from build123d import *

# Parameters (mm, degrees)
SKETCH1_R                       = 12.7
BOSS_EXTRUDE1_DEPTH             = 80
TAP_DRILL_FOR_1_4_20_TAP1_D     = 5.1054
TAP_DRILL_FOR_1_4_20_TAP1_DEPTH = 7.62
TAP_DRILL_FOR_1_4_20_TAP1_TIP   = 1.533816902
TAP_DRILL_FOR_1_4_20_TAP2_D     = 5.1054
TAP_DRILL_FOR_1_4_20_TAP2_DEPTH = 7.62
TAP_DRILL_FOR_1_4_20_TAP2_TIP   = 1.533816902


with BuildPart() as part:
    # Sketch1 → Boss-Extrude1 (new body)
    with BuildSketch(Plane(origin=(0, 0, 0), x_dir=(1, 0, 0), z_dir=(0, 1, 0))):
        with Locations(Location((0, 0, 0), (0, 0, 270))):
            Circle(SKETCH1_R)
    extrude(amount=BOSS_EXTRUDE1_DEPTH)

    # Tap Drill for 1/4-20 Tap1
    with Locations(Plane.XZ):
        with Locations((0, 0)):
            Hole(TAP_DRILL_FOR_1_4_20_TAP1_D / 2, depth=TAP_DRILL_FOR_1_4_20_TAP1_DEPTH)
            with Locations((0, 0, -(TAP_DRILL_FOR_1_4_20_TAP1_DEPTH + TAP_DRILL_FOR_1_4_20_TAP1_TIP / 2))):  # 118° drill point
                Cone(0, TAP_DRILL_FOR_1_4_20_TAP1_D / 2, TAP_DRILL_FOR_1_4_20_TAP1_TIP, mode=Mode.SUBTRACT)

    # Tap Drill for 1/4-20 Tap2
    with Locations(Plane(origin=(0, 80, 0), x_dir=(1, 0, 0), z_dir=(0, 1, 0))):
        with Locations((0, 0)):
            Hole(TAP_DRILL_FOR_1_4_20_TAP2_D / 2, depth=TAP_DRILL_FOR_1_4_20_TAP2_DEPTH)
            with Locations((0, 0, -(TAP_DRILL_FOR_1_4_20_TAP2_DEPTH + TAP_DRILL_FOR_1_4_20_TAP2_TIP / 2))):  # 118° drill point
                Cone(0, TAP_DRILL_FOR_1_4_20_TAP2_D / 2, TAP_DRILL_FOR_1_4_20_TAP2_TIP, mode=Mode.SUBTRACT)


solid = part.part
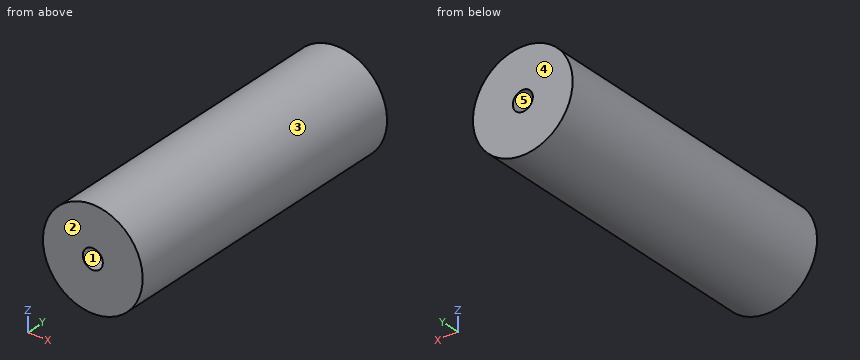
Verification items for the finished model (mm, model axes). Face numbers are marked on the shaded views. A direction names the side the tool comes from. Give positions to 0.01 mm unless a question says otherwise; leave off trailing zeros. Order: outer loops, then holes, each group sorted by start corner. A loop starts at its lowest first (then second) coordinate and runs counter-clockwise, first axis right, second up. Notation, with made-up numbers: M -6.5,84 L 8.5,84 A25 cw 8.5,103 Z; hole C 5.5,68.5 d6. An arc over 180 degrees is marked long. Use one line per item in the form item = value. Start each with the question number.
Q1. Access from +Z, -Z, +X, -X, +Y, -Y to the whole of each face (thin tool, end or side, straight path). Record for the marked faces 1 and 2.
Q2. Section check C-C (z = -10.75). Enter the section's corners in (x, y).
Q3. Go/stop test with flat-tipped pins: pin 1 Ø3 at (x, y) = (3, 55.5) entering from -Z; pin 2 Ø4 at (x, y) = (-9.5, 41) entering from -Z; pin 3 Ø12 at (y, z) = (47, 7.5) entering from -X. Record where each tip stops, or that it passes through.
Q4. Section check A-A (y = 64). Enter the section's corners in (x, z), then the cut area to 3 significant figures.
Q5. Section check B-B (x = -10.25). Enter the section's corners in (y, z), then the cut area to 3 significant figures.
Q6. Scan lines: line 1 along X through (y, z) = (4.5, 0); line 2 along Z through (x, y) = (-1, 74.5); line 3 along Z through (x, y) = (2.75, 21.5). Record each from-to range of solid material in increasing order. Write a range as [from, to].
Q7. Mould release check, pull along X, two halves, no side actions. Record for the marked faces 3, 4 and 5: +X half, -X half, draft (parallel to the pull), parting line (faces both ways), or undercut.
Evaluation:
q1.face_1 = -Y
q1.face_2 = +Z, -Z, +X, -X, -Y
q2.outline = M -6.76,0 L 6.76,0 L 6.76,80 L -6.76,80 Z
q3.pin_1 = -12.61
q3.pin_2 = -10.25
q3.pin_3 = -12.61
q4.outline = C 0,0 d25.4
q4.area = 507 mm2
q5.outline = M 0,-7.5 L 80,-7.5 L 80,7.5 L 0,7.5 Z
q5.area = 1,200 mm2
q6.line_1 = [-12.7, -2.55], [2.55, 12.7]
q6.line_2 = [-12.66, -2.35], [2.35, 12.66]
q6.line_3 = [-12.4, 12.4]
q7.face_3 = parting line
q7.face_4 = draft
q7.face_5 = undercut
